from build123d import *

# Parameters (mm, degrees)
F0_R     = 5
F1_DEPTH = 10
F2_R     = 2
F3_DEPTH = 5
F4_R     = 1.25
F5_DEPTH = 5


with BuildPart() as f1:
    # F0 (on Top) → F1 (new body)
    with BuildSketch(Plane.XY):
        Polygon((0, 5), (0, 0), (50, 0), (50, 5), (40, 5), (-10, 75), (-20, 75), (10, 5), align=None)
        with Locations((10, 30.5684879422)):
            Circle(F0_R, mode=Mode.SUBTRACT)
    extrude(amount=F1_DEPTH)

    # F2 (on face) → F3 (cut)
    with BuildSketch(Plane.XZ):
        with Locations((45, 5)):
            Circle(F2_R)
        with Locations((5, 5)):
            Circle(F2_R)
    extrude(amount=-F3_DEPTH, mode=Mode.SUBTRACT)

    # F4 (on face) → F5 (cut)
    with BuildSketch(Plane(origin=(0, 75, 0), x_dir=(-1, 0, 0), z_dir=(0, 1, 0))):
        with Locations((15, 5)):
            Circle(F4_R)
    extrude(amount=-F5_DEPTH, mode=Mode.SUBTRACT)


solid = f1.part
Design review of the part built by this model. Coordinates are the model's own, in mm. A direction names the side the tool comes from. Round coordinates to 2 decimals unless told otherwise and drop trailing zeros. Write each loop counter-clockwise with the first axis right and the second up, starting at its lowest first coordinate (ties: lowest second). Pieces come first, ordered by that corner, then holes. Notation, with made-up numbers: (35.25, 38) - (82.25, 38) arc R34 cw to (82.25, 71) - close; hole circle Ø3 at (-11.5, 42). An arc over 180 degrees is marked (long way). Return JSON: item names as keys, results as strings. Group by question number.
Item 1: Insertion check: P1, Ø1, axis at y = 49, z = 3.5, coming from the -X side; P2, Ø1.2, axis at x = -14.5, z = 5, coming from the +Y side; P3, Ø3, axis at x = 5, z = 5, coming from the -Y side. Each pin has a flat end and moves straight along its axis. Give the tip position at first contact, or say it passes through.
Item 2: The part is to be moulded in two halves that separate along Y. For faces 1 (the face through (-15, 70, 5)), 2 (the face through (-5, 40, 5)), 3 (the face through (3, 2, 5)), 4 (the face through (12.307, 26.133, 4.93)), say which applies: pulls with the +Y half, pulls with the -Y half, needs draft (parallel to the pull), parting line crosses it, or undercut.
Item 3: For probe 1 along Y at (x, z) = (43, 3.5); probe 2 along X at (y, z) = (4, 6.5); probe 3 along Y at (x, z) = (2.5, 2.75), list the stretches that pass through material, from the lowest coordinate up. Write a range as [from, to].
Item 4: We need section B-B on z = 5. Write out the cut boundary in (x, y), and give its area (3 significant figures).
Item 5: We need section A-A on x = 45. Write out the cut boundary in (y, z), and give its area (3 significant figures).
Item 6: We need section C-C on x = 18. Write out the cut boundary in (y, z).
Item 7: Machinability: for faces 5 (the face through (42.8, 5, 4.9)), 6 (the face through (2.8, 5, 4.9)), 7 (the face through (-14.73, 72.54, 3.78)), which of the approach directions +Z, -Z, +X, -X, +Y, -Y give a long, thin tool a straight path to every point of the face, cutting with its end or side? Answer none if there is none.
Item 8: We need section D-D on y = 43.5. Write out the cut boundary in (x, z), and give its area (3 significant figures).
Model answer:
{
 "1": {"P1": "stops at x = -9.07", "P2": "stops at y = 70", "P3": "stops at y = 13.17"},
 "2": {"face 1": "pulls with the +Y half", "face 2": "undercut", "face 3": "needs draft", "face 4": "undercut"},
 "3": {"probe 1": "y = [0, 5]", "probe 2": "x = [0, 3.68], [6.32, 43.68], [46.32, 50]", "probe 3": "y = [0, 5], [22.5, 57.5]"},
 "4": {"outline": "(-20, 75) - (10, 5) - (7, 5) - (7, 0) - (43, 0) - (43, 5) - (40, 5) - (-10, 75) - (-13.75, 75) - (-13.75, 70) - (-16.25, 70) - (-16.25, 75) - close; (0, 0) - (3, 0) - (3, 5) - (0, 5) - close; (47, 0) - (50, 0) - (50, 5) - (47, 5) - close; hole circle Ø10 at (10, 30.57)", "area": "1,520 mm²"},
 "5": {"outline": "(0, 0) - (5, 0) - (5, 3) - (0, 3) - close; (0, 7) - (5, 7) - (5, 10) - (0, 10) - close", "area": "30.0 mm²"},
 "6": {"outline": "(0, 0) - (35.8, 0) - (35.8, 10) - (0, 10) - close"},
 "7": {"face 5": "+Z, -Z, +X, +Y", "face 6": "+Z, -Z, -X", "face 7": "+Y"},
 "8": {"outline": "(-6.5, 0) - (12.5, 0) - (12.5, 10) - (-6.5, 10) - close", "area": "190 mm²"}
}
